The model under review builds one solid part; all positions refer to its coordinate system, in mm. A direction names the side the tool comes from. Coordinates: 2 decimals unless noted, no trailing zeros. Loops run counter-clockwise (first coordinate to the right, second up) from the corner with the lowest first, then second, coordinate; pieces in that order, holes last. Notation, with made-up numbers: M -4,3 L 45,3 A9 cw 45,18 Z; hole C -15.5,0 d2. An arc over 180 degrees is marked long. Use CSV: the item, a comma, the result in double quotes. Start each with the question number.
1. For L1, parallel to Z at x = 4.75, y = 21; L2, parallel to Y at x = 4.75, z = 16; L3, parallel to Y at x = 2, z = 93.5, list the stretches that pass through material, from the lowest coordinate up.
2. Add section A-A, the plane y = 52. Write out the cut boundary in (x, z), then the cut area to 3 significant figures.
3. Add section D-D, the plane x = 1.25. State how many separate pieces and enclosed holes the cut face has, then the cut area to 3 significant figures.
4. Draft analysis for pull direction Y (two halves, no side actions). For faces 1 (the flat face through (2.958, -19.122, 91.403)), 2 (the flat face through (3, 16, 86)), 3 (the flat face through (2.958, 51.686, 92.841)), state which applies: +Y half, -Y half, draft (parallel to the pull), parting line (faces both ways), or undercut.
5. Clearance check with flat-ended pins moving along their axes: P1, Ø1.8, axis at x = 2, z = 16, coming from the +Y side; P2, Ø2.5, axis at x = 0.5, y = 48, coming from the -Z side; P3, Ø2, axis at x = 3, y = -70.5, coming from the +Z side. State where each tip first meets the part, or that it passes through.
6. Add section C-C, the plane y = -10.5. Write out the cut boundary in (x, z), then the cut area to 3 significant figures.
7. Tool access review of faces 4 (the flat face through (2.96, -59.47, 9.37)), 5 (the flat face through (3, 13, 6)), 6 (the flat face through (2.96, -68.74, 1.36)): name each direction out of +Z, -Z, +X, -X, +Y, -Y from which nothing blocks a thin tool from reaching the whole face with its end or side.
8. Add section B-B, the plane z = 169.5. Write out the cut boundary in (x, y), then the cut area to 3 significant figures.
from build123d import *

# Parameters (mm, degrees)
F1_DEPTH = 6
F2_W     = 5.8
F2_H     = 3.1
F3_DEPTH = 25
F5_DEPTH = 80.8
F7_DEPTH = 80.8
F9_DEPTH = 80.8
F10_R    = 4


with BuildPart() as f1:
    # F0 (on Right) → F1 (new body)
    with BuildSketch(Plane.YZ):
        Polygon((-75, 3.6397023427), (-65, 0), (75, 0), (75, 6), (26.9445243494, 185), (14.9445243494, 185), (-50.2061475843, 6), (-69, 12.8404028665), (-69, 20), (-75, 20), align=None)
        Polygon((68.7875391018, 6), (-43.8210809494, 6), (-14.7034622081, 86), (47.3102315485, 86), align=None, mode=Mode.SUBTRACT)
        Polygon((-12.5196408025, 92), (17.6898886416, 175), (23.4167268954, 175), (45.699433482, 92), align=None, mode=Mode.SUBTRACT)
    extrude(amount=F1_DEPTH)

    # F2 (on face) → F3 (cut)
    with BuildSketch(Plane.YZ.offset(6)):
        with Locations((-27.9, 1.55)):
            Rectangle(F2_W, F2_H)
        with Locations((47.1, 1.55)):
            Rectangle(F2_W, F2_H)
        Polygon((-5.4699128373, 128.9117947988), (-7.4536296686, 123.4615775982), (-4.5405825441, 122.4013151539), (-2.5568657128, 127.8515323545), align=None)
        Polygon((-31.1214235867, 58.4348482399), (-33.105140418, 52.9846310393), (-30.1920932936, 51.924368595), (-28.2083764623, 57.3745857955), align=None)
        Polygon((59.0417662259, 53.4862587999), (62.0357488529, 54.290042371), (60.5318957199, 59.8916872861), (57.5379130928, 59.0879037149), align=None)
        Polygon((39.5953895053, 125.9213223564), (42.5893721323, 126.7251059276), (41.0855189992, 132.3267508426), (38.0915363722, 131.5229672715), align=None)
    extrude(amount=-F3_DEPTH, mode=Mode.SUBTRACT)

    # F4 (on face) → F5 (join, through all)
    with BuildSketch(Plane(origin=(0, 13.1563663869, 36.14681957), x_dir=(1, 0, 0), z_dir=(0, 0.3420201433, 0.9396926208))):
        with BuildLine():
            ThreePointArc((2.25, -46.130467263), (3, -46.880467263), (3.75, -46.130467263))
            Line((3.75, -46.130467263), (2.25, -46.130467263))
        make_face()
    extrude(amount=F5_DEPTH)

    # F6 (on face) → F7 (join, through all)
    with BuildSketch(Plane(origin=(0, -30.8, 0), x_dir=(-1, 0, 0), z_dir=(0, 1, 0))):
        with BuildLine():
            ThreePointArc((-3.75, 3.1), (-3, 2.35), (-2.25, 3.1))
            Line((-2.25, 3.1), (-3.75, 3.1))
        make_face()
    extrude(amount=F7_DEPTH)

    # F8 (on face) → F9 (join, through all)
    with BuildSketch(Plane(origin=(0, -9.4246030822, 35.1053429162), x_dir=(1, 0, 0), z_dir=(0, -0.2592850229, 0.9658008474))):
        with BuildLine():
            Line((2.25, 70.8907736942), (3.75, 70.8907736942))
            ThreePointArc((3.75, 70.8907736942), (3, 71.6407736942), (2.25, 70.8907736942))
        make_face()
    extrude(amount=F9_DEPTH)

    # F10
    f10_edges = [f1.edges().sort_by_distance(p)[0] for p in [
        (3, -75, 3.639702),
        (3, -75, 20),
    ]]
    fillet(f10_edges, radius=F10_R)


solid = f1.part
Computed:
1,L1,"z = 0 to 6, 86 to 92, 175 to 185"
1,L2,"y = -75 to -69, -46.57 to -40.18, 66.1 to 72.32"
1,L3,"y = -18.36 to -11.97, 45.3 to 51.51"
2,outline,"M 0,0 L 6,0 L 6,6 L 0,6 Z; M 0,68.53 L 6,68.53 L 6,91.67 L 0,91.67 Z"
2,area,"175 mm^2"
3,separate pieces,"1"
3,enclosed holes,"2"
3,area,"3,560 mm^2"
4,face 1,"-Y half"
4,face 2,"undercut"
4,face 3,"+Y half"
5,P1,"stops at y = 72.56"
5,P2,"stops at z = 3.1"
5,P3,"stops at z = 20"
6,outline,"M 0,0 L 6,0 L 6,6 L 0,6 Z; M 0,86 L 6,86 L 6,92 L 0,92 Z; M 0,97.55 L 6,97.55 L 6,115.09 L 0,115.09 Z"
6,area,"177 mm^2"
7,face 4,"+Z, +X, -X"
7,face 5,"+X, -X"
7,face 6,"-Z, +X, -X, -Y"
8,outline,"M 0,9.3 L 6,9.3 L 6,15.69 L 0,15.69 Z; M 0,24.89 L 6,24.89 L 6,31.11 L 0,31.11 Z"
8,area,"75.6 mm^2"
